Source: CAD feature listing. Evaluate the final solid. Frame: model axes, mm. Give positions to 0.01 mm unless a question says otherwise; leave off trailing zeros. Order: outer loops, then holes, each group sorted by start corner. A loop starts at its lowest first (then second) coordinate and runs counter-clockwise, first axis right, second up. Notation, with made-up numbers: M 6,-16 L 55,-16 A25 ccw 55,22 Z; hole C 48.5,72 d2. An arc over 180 degrees is marked long. Return JSON: item names as keys, results as strings.
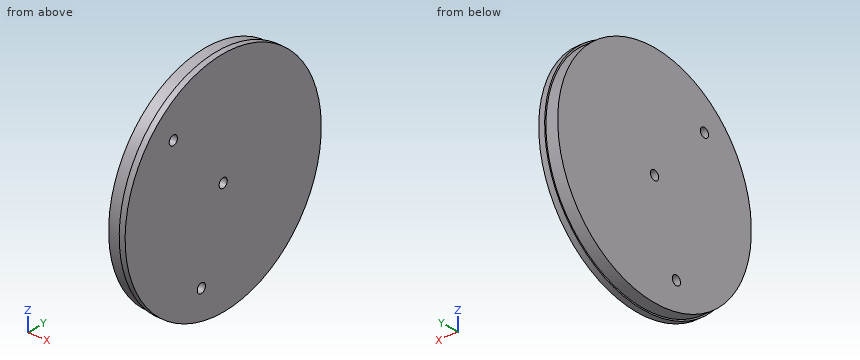
from build123d import *

# Parameters (mm, degrees)
SKETCH1_R           = 76.2
BOSS_EXTRUDE1_DEPTH = 12
SKETCH2_OUTSIDE_W   = 197.572
SKETCH2_OUTSIDE_H   = 197.572
SKETCH2_OUTSIDE_R   = 75.2221
CUT_EXTRUDE1_DEPTH  = 8
SKETCH3_R           = 3.175
CUT_EXTRUDE2_DEPTH  = 109.429147373
SKETCH5_R           = 3.175
CUT_EXTRUDE3_DEPTH  = 109.429147373
CIRPATTERN1_COUNT   = 3


with BuildPart() as part:
    # Sketch1 → Boss-Extrude1 (new body)
    with BuildSketch(Plane(origin=(0, 0, 0), x_dir=(0, 0, -1), z_dir=(1, 0, 0))):
        Circle(SKETCH1_R)
    extrude(amount=BOSS_EXTRUDE1_DEPTH)

    # Sketch2 outside → Cut-Extrude1 (cut)
    with BuildSketch(Plane.ZY):
        Rectangle(SKETCH2_OUTSIDE_W, SKETCH2_OUTSIDE_H)
        Circle(SKETCH2_OUTSIDE_R, mode=Mode.SUBTRACT)
    extrude(amount=-CUT_EXTRUDE1_DEPTH, mode=Mode.SUBTRACT)

    # Sketch3 → Cut-Extrude2 (cut, through all)
    with BuildSketch(Plane(origin=(12, 0, 0), x_dir=(0, 0, -1), z_dir=(1, 0, 0))):
        Circle(SKETCH3_R)
    extrude(amount=-CUT_EXTRUDE2_DEPTH, mode=Mode.SUBTRACT)

    # Sketch5 → Cut-Extrude3 (cut, through all)
    with BuildSketch(Plane(origin=(12, 0, 0), x_dir=(0, 0, -1), z_dir=(1, 0, 0))):
        with Locations((-41.99401686, -38.763707871)):
            Circle(SKETCH5_R)
    cut_extrude3 = extrude(amount=-CUT_EXTRUDE3_DEPTH, mode=Mode.SUBTRACT)

    # CirPattern1: Cut-Extrude3 ×3 about axis, 1 skipped
    cirpattern1_axis = Axis((12, 0, 0), (1, 0, 0))
    add([cut_extrude3.rotate(cirpattern1_axis, i * 360 / CIRPATTERN1_COUNT) for i in range(1, CIRPATTERN1_COUNT) if i not in (2,)], mode=Mode.SUBTRACT)


solid = part.part
1. Section query D-D (y = 52). Return loops of the section in (x, z).
Evaluation:
{"outline": "M 0,-54.35 L 8,-54.35 L 8,-55.7 L 12,-55.7 L 12,55.7 L 8,55.7 L 8,54.35 L 0,54.35 Z"}
2. Section query C-C (z = -32.5). Return loops of the section in (x, y).
Evaluation:
{"outline": "M 0,-67.84 L 8,-67.84 L 8,-68.92 L 12,-68.92 L 12,68.92 L 8,68.92 L 8,67.84 L 0,67.84 Z"}
3. First-contact query: pin 1 (4 mm diameter, centred on x = 7, z = -5.5, fed in from -Y); pin 2 (4 mm diameter, centred on x = 9, z = 35, fed in from -Y). Flat tips, straight axial feed; report the tip coordinate or a pass-through.
Evaluation:
{"pin 1": "stops at y = -76.11", "pin 2": "stops at y = -68.68"}
4. Section query A-A (y = 0). Return loops of the section in (x, z) (3 decimals), then the cut area to 3 significant figures.
Evaluation:
{"outline": "M 0,-75.222 L 8,-75.222 L 8,-76.2 L 12,-76.2 L 12,-3.175 L 0,-3.175 Z; M 0,3.175 L 12,3.175 L 12,76.2 L 8,76.2 L 8,75.222 L 0,75.222 Z", "area": "1,740 mm^2"}
5. Ray query, probe 1 along Y at (x, z) = (3.25, 0) (3 decimals); probe 2 along Z at (x, y) = (5.75, -37); probe 3 along Y at (x, z) = (3.5, -1.5). Return the intervals inside material, ascending.
Evaluation:
{"probe 1": "y = -75.222 to -3.175, 3.175 to 75.222", "probe 2": "z = -65.49 to 39.35, 44.63 to 65.49", "probe 3": "y = -75.21 to -2.8, 2.8 to 75.21"}
